For this review, take the finished solid that the model builds, in its own axes (mm). Give positions to 0.01 mm unless a question says otherwise; leave off trailing zeros. Loops run counter-clockwise (first coordinate to the right, second up) from the corner with the lowest first, then second, coordinate; pieces in that order, holes last. Notation, with made-up numbers: (-33.75, -7) - (-16.75, -7) arc R7 ccw to (-16.75, 6) - close; hole circle Ø3 at (47.25, 74). An arc over 180 degrees is marked (long way). Put each result on its own line as item: value.
from build123d import *

# Parameters (mm, degrees)
BOSS_EXTRUDE1_DEPTH  = 2.54
SKETCH2_W            = 107.95
SKETCH2_H            = 63.5
CUT_EXTRUDE1_DEPTH   = 238.771783963
CUT_EXTRUDE4_START   = -2.54
CUT_EXTRUDE4_DEPTH   = 2.54
SKETCH4_R            = 4.7625
SKETCH4_R_2          = 6.35
SKETCH4_R_3          = 10.5
CUT_EXTRUDE3_DEPTH   = 238.771784093
M6_CLEARANCE_HOLE1_D = 7
M4_CLEARANCE_HOLE1_D = 4.8


with BuildPart() as part:
    # Sketch1 → Boss-Extrude1 (new body)
    with BuildSketch(Plane(origin=(0, 0, 0), x_dir=(1, 0, 0), z_dir=(0, 1, 0))):
        with BuildLine():
            Line((222.25, -14.612459999), (222.25, 36.187540001))
            Line((222.25, 36.187540001), (-222.25, 36.187540001))
            Line((-222.25, 36.187540001), (-222.25, -14.612459999))
            ThreePointArc((-222.25, -14.612459999), (-201.791408666, -64.003868664), (-152.4, -84.462459999))
            Line((-152.4, -84.462459999), (152.4, -84.462459999))
            ThreePointArc((152.4, -84.462459999), (201.791408666, -64.003868664), (222.25, -14.612459999))
        make_face()
    extrude(amount=BOSS_EXTRUDE1_DEPTH)

    # Sketch2 → Cut-Extrude1 (cut, through all)
    with BuildSketch(Plane(origin=(0, 2.54, 0), x_dir=(1, 0, 0), z_dir=(0, 1, 0))):
        with Locations((0, -42.552459999)):
            Rectangle(SKETCH2_W, SKETCH2_H)
    extrude(amount=-CUT_EXTRUDE1_DEPTH, mode=Mode.SUBTRACT)

    # Sketch5 → Cut-Extrude4 (cut)
    with BuildSketch(Plane(origin=(0, 2.54, 0), x_dir=(1, 0, 0), z_dir=(0, 1, 0)).offset(CUT_EXTRUDE4_START)):
        with BuildLine():
            ThreePointArc((-222.25, -14.612459999), (-218.970589391, -35.763798683), (-209.440289817, -54.929055063))
            add(Edge.make_bspline(
                [(-209.440289817, -54.929055063), (-204.823931799, -55.506078622), (-202.304901657, -25.266816537), (-219.26819847, -8.373976847), (-222.25, -8.829558466)],
                knots=[0, 0, 0, 0, 0.32580352, 0.516674914, 0.516674914, 0.516674914, 0.516674914], degree=3))
            Line((-222.25, -8.829558466), (-222.25, -14.612459999))
        make_face()
        with BuildLine():
            add(Edge.make_bspline(
                [(-222.25, -8.829558466), (-229.800526338, -9.983183543), (-216.288594077, -54.073048471), (-209.440289817, -54.929055063)],
                knots=[0.516674914, 0.516674914, 0.516674914, 0.516674914, 1, 1, 1, 1], degree=3))
            ThreePointArc((-209.440289817, -54.929055063), (-218.970589391, -35.763798683), (-222.25, -14.612459999))
            Line((-222.25, -14.612459999), (-222.25, -8.829558466))
        make_face()
        with BuildLine():
            add(Edge.make_bspline(
                [(209.440289817, -54.929055063), (204.823931799, -55.506078622), (202.304901657, -25.266816537), (235.136564978, 7.428480335), (216.288594077, -54.073048471), (209.440289817, -54.929055063)],
                knots=[0, 0, 0, 0, 0.32580352, 0.516674914, 1, 1, 1, 1], degree=3))
        make_face()
    extrude(amount=CUT_EXTRUDE4_DEPTH, mode=Mode.SUBTRACT)

    # Sketch4 → Cut-Extrude3 (cut, through all)
    with BuildSketch(Plane(origin=(0, 2.54, 0), x_dir=(1, 0, 0), z_dir=(0, 1, 0))):
        with Locations(Location((171.45, 15.867540001, 0), (0, 0, 270))):
            Circle(SKETCH4_R)
        with Locations(Location((-139.7, 4.437540001, 0), (0, 0, 270))):
            Circle(SKETCH4_R_2)
        with Locations(Location((127, 17.137540001, 0), (0, 0, 270))):
            Circle(SKETCH4_R_2)
        with Locations(Location((127, -14.612459999, 0), (0, 0, 270))):
            Circle(SKETCH4_R_2)
        with Locations(Location((171.45, -14.612459999, 0), (0, 0, 270))):
            Circle(SKETCH4_R)
        with Locations(Location((-177.8, -40.012459999, 0), (0, 0, 270))):
            Circle(SKETCH4_R_3)
        with Locations(Location((-177.8, 4.437540001, 0), (0, 0, 270))):
            Circle(SKETCH4_R_3)
        with Locations(Location((-107.95, 4.437540001, 0), (0, 0, 270))):
            Circle(SKETCH4_R_2)
        with BuildLine():
            Line((-140.55, -48.067737772), (-140.55, -49.812459999))
            Line((-140.55, -49.812459999), (-138.85, -49.812459999))
            Line((-138.85, -49.812459999), (-138.85, -48.067737772))
            ThreePointArc((-138.85, -48.067737772), (-139.7, -31.912459999), (-140.55, -48.067737772))
        make_face()
        with BuildLine():
            Line((153.9875, -52.712459999), (144.4625, -52.712459999))
            ThreePointArc((144.4625, -52.712459999), (149.225, -38.424959999), (153.9875, -52.712459999))
        make_face()
    extrude(amount=-CUT_EXTRUDE3_DEPTH, mode=Mode.SUBTRACT)

    # M6 Clearance Hole1 (through all)
    with Locations(Plane.XZ):
        with Locations((92.075, -20.32), (200.025000005, 14.612459999), (98.425, 72.39), (-92.075, -20.32), (-200.025000005, 14.612459999), (-98.425, 72.39)):
            Hole(M6_CLEARANCE_HOLE1_D / 2)

    # M4 Clearance Hole1 (through all)
    with Locations(Plane(origin=(0, 2.54, 0), x_dir=(1, 0, 0), z_dir=(0, 1, 0))):
        with Locations((-78.7827, -75.5731381), (-79, -28.2331381), (-38.130967929, 17.4595619), (38.130967929, 17.4595619), (79, -28.2331381), (78.7827, -75.5731381)):
            Hole(M4_CLEARANCE_HOLE1_D / 2)


solid = part.part
1) Take a section at C-C on z = -6. State the section outline as (x, y) points.
Geometry check:
outline: (-222.25, 0) - (-188.18, 0) - (-188.18, 2.54) - (-222.25, 2.54) - close; (-167.42, 0) - (-145.85, 0) - (-145.85, 2.54) - (-167.42, 2.54) - close; (-133.55, 0) - (-114.1, 0) - (-114.1, 2.54) - (-133.55, 2.54) - close; (-101.8, 0) - (222.25, 0) - (222.25, 2.54) - (-101.8, 2.54) - close
2) Take a section at A-A on x = -15.5. State the section outline as (y, z) points.
Geometry check:
outline: (0, -36.19) - (2.54, -36.19) - (2.54, 10.8) - (0, 10.8) - close; (0, 74.3) - (2.54, 74.3) - (2.54, 84.46) - (0, 84.46) - close
3) Insertion check: pin 1 Ø7.5 at (x, z) = (171.45, 14.61) entering from -Y; pin 2 Ø0.5 at (y, z) = (1, 49) entering from -X. Each pin has a flat end and moves straight along its axis. Give the tip position at first contact, or say it passes through.
Geometry check:
pin 1: passes through
pin 2: stops at x = -205.88
4) Take a section at D-D on y = 1.95. State how many separate pieces and enclosed holes the cut face has, and give its area (3 significant figures).
Geometry check:
separate pieces: 1
enclosed holes: 23
area: 41,700 mm²
5) Wall thickness on line 1 (X direction, y = 0.2, z = 40) (3 decimals); line 2 (Z direction, x = 126.5, y = 1.5); line 3 (Z direction, x = 19, y = 2.35): over which ranges is each line inside the solid? List them lowest first.
Geometry check:
line 1: x = -205.428 to -188.3, -167.3 to -147.8, -131.6 to -53.975, 53.975 to 144.479, 153.971 to 205.428
line 2: z = -36.19 to -23.47, -10.81 to 8.28, 20.94 to 84.46
line 3: z = -36.19 to 10.8, 74.3 to 84.46
6) Take a section at B-B on x = 127. State the section outline as (y, z) points.
Geometry check:
outline: (0, -36.19) - (2.54, -36.19) - (2.54, -23.49) - (0, -23.49) - close; (0, -10.79) - (2.54, -10.79) - (2.54, 8.26) - (0, 8.26) - close; (0, 20.96) - (2.54, 20.96) - (2.54, 84.46) - (0, 84.46) - close
7) Draft analysis for pull direction X (two halves, no side actions). For faces 1 (the face through (95.57, 1.29, -20.17)), 2 (the face through (-3, 0, 10)), 3 (the face through (184.101, 1.252, 76.855)), state which applies: pulls with the +X half, pulls with the -X half, needs draft (parallel to the pull), parting line crosses it, or undercut.
Geometry check:
face 1: undercut
face 2: needs draft
face 3: pulls with the +X half
